The model under review builds one solid part; all positions refer to its coordinate system, in mm. Face numbers are marked on the shaded views. Give positions to 0.01 mm unless a question says otherwise; leave off trailing zeros. Write each loop counter-clockwise with the first axis right and the second up, starting at its lowest first coordinate (ties: lowest second). Pieces come first, ordered by that corner, then holes. Notation, with made-up numbers: (37, -16.5) - (86, -16.5) arc R18 cw to (86, -4.5) - close; hole circle Ø10 at (27, 63). An arc over 180 degrees is marked (long way). Write item = value, one per line.
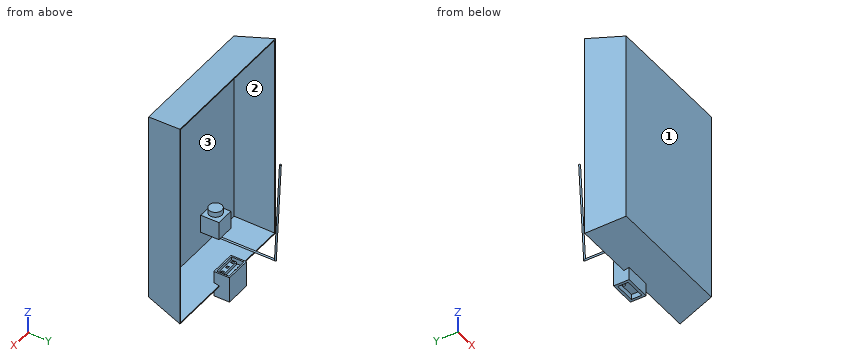
```python
from build123d import *

# Parameters (mm, degrees)
SKETCH2_W           = 250
SKETCH2_H           = 370
SKETCH1_W           = 280
SKETCH1_H           = 400
SHELL1_T            = -2
SKETCH3_W           = 50
SKETCH3_H           = 50
CUT_EXTRUDE1_DEPTH  = 10
SKETCH4_W           = 50
SKETCH4_H           = 50
BOSS_EXTRUDE2_DEPTH = 30
SKETCH6_W           = 44
SKETCH6_H           = 24
CUT_EXTRUDE2_DEPTH  = 10
SKETCH7_W           = 40
SKETCH7_H           = 20
CUT_EXTRUDE3_DEPTH  = 10
SKETCH8_R           = 2.5
CUT_EXTRUDE4_DEPTH  = 60
SKETCH9_W           = 40
SKETCH9_H           = 10
SKETCH9_W_2         = 5
SKETCH9_H_2         = 5
BOSS_EXTRUDE3_DEPTH = 6
SKETCH10_W          = 35
SKETCH10_H          = 35
BOSS_EXTRUDE5_DEPTH = 35
SKETCH11_R          = 12.5
BOSS_EXTRUDE6_DEPTH = 10
SWEEP1_PROFILE_R    = 1.5


with BuildPart() as part:
    # Sketch2 → Loft1 section 0
    with BuildSketch(Plane(origin=(0, -70, 0), x_dir=(1, 0, 0), z_dir=(0, 1, 0))):
        Rectangle(SKETCH2_W, SKETCH2_H)
    # Sketch1 → Loft1 section 1
    with BuildSketch(Plane(origin=(0, 0, 0), x_dir=(1, 0, 0), z_dir=(0, 1, 0))):
        Rectangle(SKETCH1_W, SKETCH1_H)
    loft()

    # Shell1
    shell1_openings = [part.faces().sort_by_distance(p)[0] for p in [
        (0, 0, 0),
    ]]
    offset(amount=SHELL1_T, openings=shell1_openings, kind=Kind.INTERSECTION)

    # Sketch3 → Cut-Extrude1 (cut)
    with BuildSketch(Plane(origin=(0, 0, 0), x_dir=(1, 0, 0), z_dir=(0, 1, 0))):
        with Locations((0, 200)):
            Rectangle(SKETCH3_W, SKETCH3_H)
    extrude(amount=-CUT_EXTRUDE1_DEPTH, mode=Mode.SUBTRACT)



with BuildPart() as body_2:
    # Sketch4 → Boss-Extrude2 (new body)
    with BuildSketch(Plane(origin=(0, -10, 0), x_dir=(1, 0, 0), z_dir=(0, 1, 0))):
        with Locations((0, 197.857142857)):
            Rectangle(SKETCH4_W, SKETCH4_H)
    extrude(amount=BOSS_EXTRUDE2_DEPTH)

    # Sketch6 → Cut-Extrude2 (cut)
    with BuildSketch(Plane.XY.offset(-172.857142857)):
        with Locations((0, 5)):
            Rectangle(SKETCH6_W, SKETCH6_H)
    extrude(amount=-CUT_EXTRUDE2_DEPTH, mode=Mode.SUBTRACT)

    # Sketch7 → Cut-Extrude3 (cut)
    with BuildSketch(Plane(origin=(0, 0, -222.857142857), x_dir=(-1, 0, 0), z_dir=(0, 0, -1))):
        with Locations((0, 5)):
            Rectangle(SKETCH7_W, SKETCH7_H)
    extrude(amount=-CUT_EXTRUDE3_DEPTH, mode=Mode.SUBTRACT)

    # Sketch8 → Cut-Extrude4 (cut)
    with BuildSketch(Plane.XY.offset(-182.857142857)):
        with Locations((-15.301608644, 11.712017977)):
            Circle(SKETCH8_R)
        with Locations((-7.133483514, 11.712017977)):
            Circle(SKETCH8_R)
    extrude(amount=-CUT_EXTRUDE4_DEPTH, mode=Mode.SUBTRACT)


with BuildPart() as part_1:
    add(part.part)

    add(body_2.part)  # Boss-Extrude3 merges body 2
    # Sketch9 → Boss-Extrude3 (add)
    with BuildSketch(Plane.XY.offset(-182.857142857)):
        with Locations((0.504671377, -0.618402812)):
            Rectangle(SKETCH9_W, SKETCH9_H)
        with Locations((-15.511503932, -0.618402812)):
            Rectangle(SKETCH9_W_2, SKETCH9_H_2, mode=Mode.SUBTRACT)
        with Locations((-0.511503932, -0.618402812)):
            Rectangle(SKETCH9_W_2, SKETCH9_H_2, mode=Mode.SUBTRACT)
        with Locations((14.488496068, -0.618402812)):
            Rectangle(SKETCH9_W_2, SKETCH9_H_2, mode=Mode.SUBTRACT)
    extrude(amount=BOSS_EXTRUDE3_DEPTH)



with BuildPart() as body_2_2:
    # Sketch10 → Boss-Extrude5 (new body)
    with BuildSketch(Plane(origin=(0, -68, 0), x_dir=(1, 0, 0), z_dir=(0, 1, 0))):
        with Locations((-42.39654967, 133.244997545)):
            Rectangle(SKETCH10_W, SKETCH10_H)
    extrude(amount=BOSS_EXTRUDE5_DEPTH)


with BuildPart() as part_2:
    add(part_1.part)

    add(body_2_2.part)  # Boss-Extrude6 merges body 2 2
    # Sketch11 → Boss-Extrude6 (add)
    with BuildSketch(Plane.XY.offset(-115.744997545)):
        with Locations(Location((-43.843818636, -51.947268965, 0), (0, 0, 180))):  # turned: the seam where the file's is
            Circle(SKETCH11_R)
    extrude(amount=BOSS_EXTRUDE6_DEPTH)

    # Sweep1: sweep along a path in Sketch12
    with BuildLine(Plane.ZY.offset(34.89654967)) as sweep1_path:
        Line((-149.877541463, -51.005012101), (-154.877541463, -51.005012101))
        Line((-154.877541463, -51.005012101), (-154.877541463, 68.994987899))
        Line((-154.877541463, 68.994987899), (44.889790726, 78.639312125))
    # Sweep1 profile (on start of the path) → Sweep1 (sweep)
    with BuildSketch(Plane(origin=(-34.89654967, -51.005012101, -149.877541463), x_dir=(0, -1, 0), z_dir=(0, 0, -1))):
        Circle(SWEEP1_PROFILE_R)
    sweep(path=sweep1_path.line, transition=Transition.RIGHT)


solid = part_2.part
```
1. Take a section at A-A on z = -191. Count the separate pieces of the cut face and the enclosed holes in it, and give its area (3 significant figures).
Findings below:
separate_pieces = 2
enclosed_holes = 2
area = 4,110 mm²
2. Insertion check: P1, Ø11, axis at x = 0.5, z = -219.5, coming from the +Y side; P2, Ø1.5, axis at x = 15, y = -2, coming from the +Z side; P3, Ø1, axis at x = -110, y = -11, coming from the -Z side. Each pin has a flat end and moves straight along its axis. Give the tip position at first contact, or say it passes through.
Findings below:
P1 = 20
P2 = 199.73
P3 = -197.75
3. Take a section at C-C on y = 43.5. Give the boundary of the cut face in (x, z), and give its area (3 significant figures).
Findings below:
outline = circle Ø3 at (-34.9, -154.88)
area = 7.07 mm²
4. For line 1 (Y direction, x = -56.5, z = 120); line 2 (X direction, y = -10, z = -74); line 3 (X direction, y = -52.5, z = 164.5), list the stretches that pass through material, from the lowest coordinate up. Write a range as from..to.
Findings below:
line_1 = -70..-68
line_2 = -137.86..-135.81, 135.81..137.86
line_3 = -128.75..-126.7, 126.7..128.75
5. Draft analysis for pull direction X (two halves, no side actions). For the marked faces 1, 2 and 3, state which applies: +X half, -X half, draft (parallel to the pull), parting line (faces both ways), or undercut.
Findings below:
face_1 = draft
face_2 = undercut
face_3 = undercut
